Part print with two shaded views. Sizes in mm from the minimum x, y, z corner. A direction names the side the tool comes from. Round coordinates to 2 decimals unless told otherwise and drop trailing zeros. Loops run counter-clockwise (first coordinate to the right, second up) from the corner with the lowest first, then second, coordinate; pieces in that order, holes last. Notation, with made-up numbers: (88.25, -33.75) - (122.25, -33.75) arc R17 ccw to (122.25, -20.75) - close; hole circle Ø1 at (-6.75, 9.5). An arc over 180 degrees is marked (long way). One line per question, with ' | ' between items.
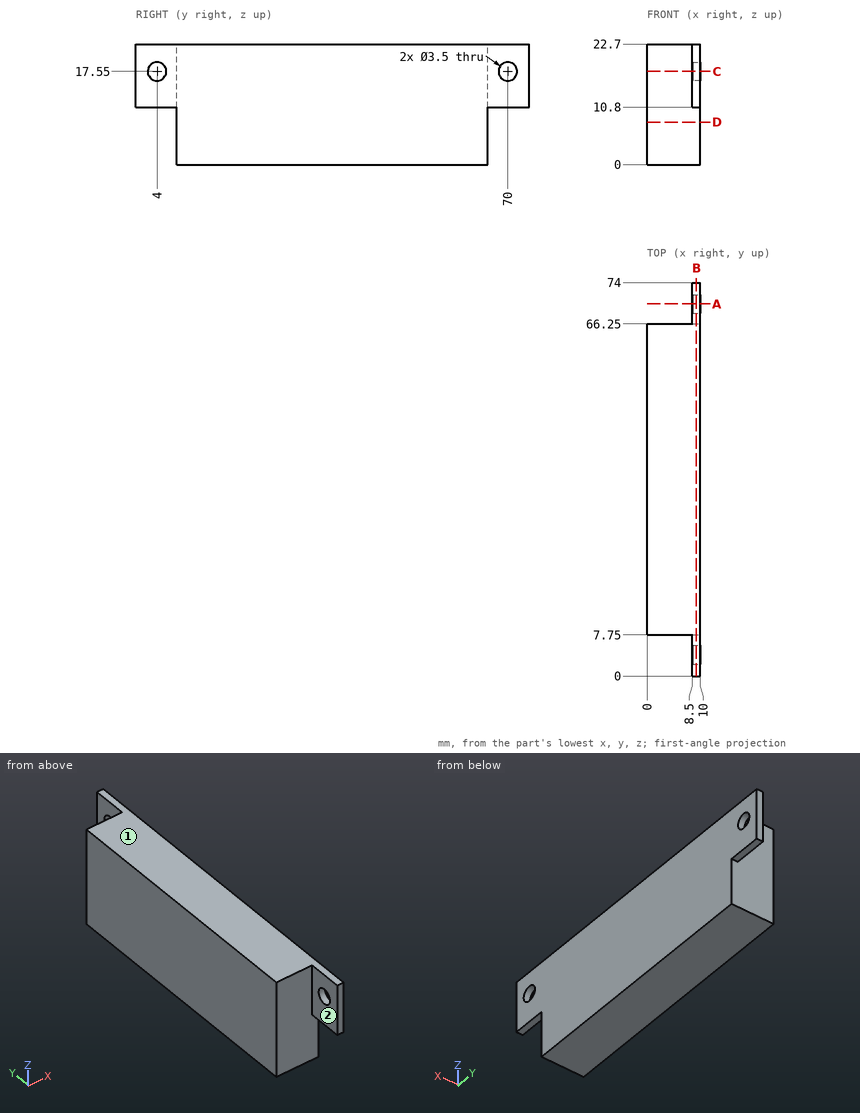
(1) Probe L1, parallel to Y at x = 9.1, z = 17.55; L2, parallel to Z at x = 9.4, y = 70; L3, parallel to Y at x = 7.5, z = 13.75. List the from-to ranges inside material, lowest first.
Results found:
L1: y = 0 to 2.25, 5.75 to 68.25, 71.75 to 74 | L2: z = 10.8 to 15.8, 19.3 to 22.7 | L3: y = 7.75 to 66.25
(2) Cut at C-C, the plane z = 17.55. Write the cut outline in (x, y).
Results found:
outline: (0, 7.75) - (8.5, 7.75) - (8.5, 5.75) - (10, 5.75) - (10, 68.25) - (8.5, 68.25) - (8.5, 66.25) - (0, 66.25) - close; (8.5, 0) - (10, 0) - (10, 2.25) - (8.5, 2.25) - close; (8.5, 71.75) - (10, 71.75) - (10, 74) - (8.5, 74) - close
(3) Drop flat-ended pins along their axis: P1, Ø4, axis at y = 69, z = 15.5, coming from the -X side; P2, Ø1.5, axis at x = 5.5, z = 12, coming from the -Y side; P3, Ø1.6, axis at x = 9, y = 68.5, coming from the -Z side. Give the stop position or say it passes through.
Results found:
P1: stops at x = 8.5 | P2: stops at y = 7.75 | P3: stops at z = 10.8
(4) Cut at A-A, the plane y = 70. Write the cut outline in (x, z).
Results found:
outline: (8.5, 10.8) - (10, 10.8) - (10, 15.8) - (8.5, 15.8) - close; (8.5, 19.3) - (10, 19.3) - (10, 22.7) - (8.5, 22.7) - close
(5) Cut at D-D, the plane z = 8. Write the cut outline in (x, y).
Results found:
outline: (0, 7.75) - (10, 7.75) - (10, 66.25) - (0, 66.25) - close
(6) Cut at B-B, the plane x = 9.25. Write the cut outline in (y, z), then the cut area to 3 significant figures.
Results found:
outline: (0, 10.8) - (7.75, 10.8) - (7.75, 0) - (66.25, 0) - (66.25, 10.8) - (74, 10.8) - (74, 22.7) - (0, 22.7) - close; hole circle Ø3.5 at (4, 17.55); hole circle Ø3.5 at (70, 17.55) | area: 1,490 mm²
(7) Tool access for the marked faces 1 and 2: list every direction of +Z, -Z, +X, -X, +Y, -Y with a clear straight run to the whole face (end or side of a thin tool).
Results found:
face 1: +Z, +X, -X, +Y, -Y | face 2: +Z, -Z, -X, -Y
